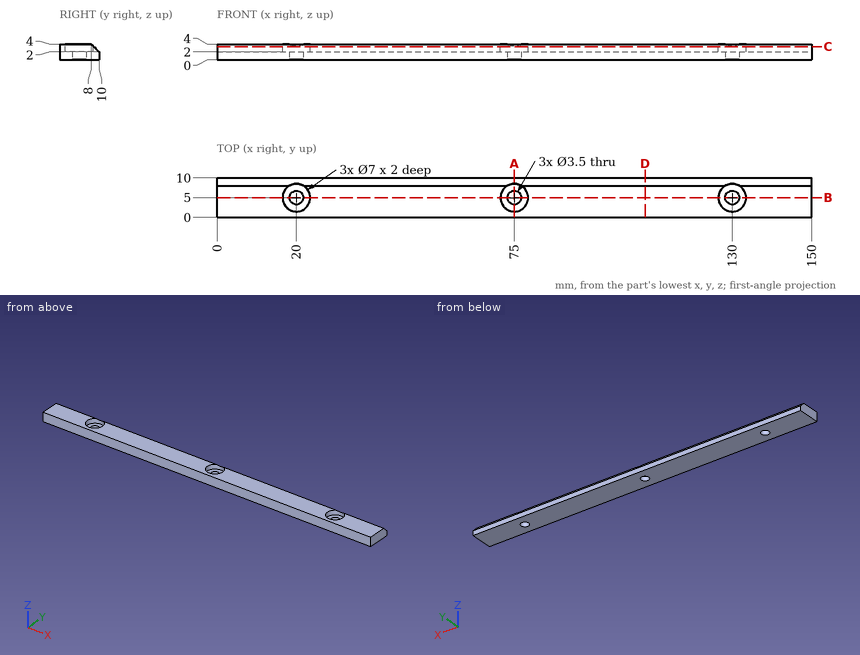
For this review, use the dimensioned drawing (mm, ordinates from the lowest corner) and the shaded views. Coordinates: 2 decimals unless noted, no trailing zeros. Loops run counter-clockwise (first coordinate to the right, second up) from the corner with the lowest first, then second, coordinate; pieces in that order, holes last.
1. Add section B-B, the plane y = 5. Give the boundary of the cut face in (x, z).
2. For line 1 (X direction, y = 5, z = 3.1); line 2 (X direction, y = 6, z = 2.55); line 3 (Y direction, x = 20, z = 1.45), list the stretches that pass through material, from the lowest coordinate up.
3. Insertion check: P1, Ø3, axis at x = 20, y = 5, coming from the -Z side; P2, Ø2, axis at x = 76, y = 5, coming from the +Z side. Each pin has a flat end and moves straight along its axis. Give the tip position at first contact, or say it passes through.
4. Add section A-A, the plane x = 75. Give the boundary of the cut face in (y, z).
5. Add section C-C, the plane z = 3.35. Give the boundary of the cut face in (x, y).
6. Add section D-D, the plane x = 108. Give the boundary of the cut face in (y, z).
Result:
1. outline: (0, 0) - (18.25, 0) - (18.25, 2) - (16.5, 2) - (16.5, 4) - (0, 4) - close; (21.75, 0) - (73.25, 0) - (73.25, 2) - (71.5, 2) - (71.5, 4) - (23.5, 4) - (23.5, 2) - (21.75, 2) - close; (76.75, 0) - (128.25, 0) - (128.25, 2) - (126.5, 2) - (126.5, 4) - (78.5, 4) - (78.5, 2) - (76.75, 2) - close; (131.75, 0) - (150, 0) - (150, 4) - (133.5, 4) - (133.5, 2) - (131.75, 2) - close
2. line 1: x = 0 to 16.5, 23.5 to 71.5, 78.5 to 126.5, 133.5 to 150
2. line 2: x = 0 to 16.65, 23.35 to 71.65, 78.35 to 126.65, 133.35 to 150
2. line 3: y = 0 to 3.25, 6.75 to 10
3. P1: passes through
3. P2: stops at z = 2
4. outline: (0, 0) - (3.25, 0) - (3.25, 2) - (1.5, 2) - (1.5, 4) - (0, 4) - close; (6.75, 0) - (10, 0) - (10, 2) - (8.5, 3.5) - (8.5, 2) - (6.75, 2) - close
5. outline: (0, 0) - (150, 0) - (150, 8.65) - (0, 8.65) - close; hole circle Ø7 at (20, 5); hole circle Ø7 at (75, 5); hole circle Ø7 at (130, 5)
6. outline: (0, 0) - (10, 0) - (10, 2) - (8, 4) - (0, 4) - close
